Model file for the job. Use its own axes, mm. Coordinates: 2 decimals unless noted, no trailing zeros. Order: outer loops, then holes, each group sorted by start corner. A loop starts at its lowest first (then second) coordinate and runs counter-clockwise, first axis right, second up. Notation, with made-up numbers: (-20, 23) -> (39, 23) arc R22 ccw to (39, 30) -> close; hole circle Ø6 at (31.25, -22.5). An arc over 180 degrees is marked (long way). Write item = value, one per line. Start each with the question number.
Q1. Cut at A-A, the plane y = 35. List the corners of the cut face in (x, z).
Q2. Cut at C-C, the plane x = 130. List the corners of the cut face in (y, z), plus the area to 3 significant figures.
Q3. Wall check: line 1 (X direction, y = 34.5, z = 0.45); line 2 (X direction, y = 31, z = 0.95); line 3 (Y direction, x = 130, z = 1.3). Give the ranges that are in metal, low to high. Write a range as from..to.
Q4. Flat gauge pins, fed straight in: pin 1 (12 mm diameter, centred on x = 40, y = 35, fed in from -Z); pin 2 (2 mm diameter, centred on x = 23, z = 2, fed in from +Y); pin 3 (2 mm diameter, centred on y = 70.5, z = 2.5, fed in from -X); pin 4 (1.2 mm diameter, centred on y = 12, z = 1, fed in from -X). Where does each tip first touch, or does it go through?
Q5. Cut at B-B, the plane z = 3.4. List the corners of the cut face in (x, y), plus the area to 3 significant figures.
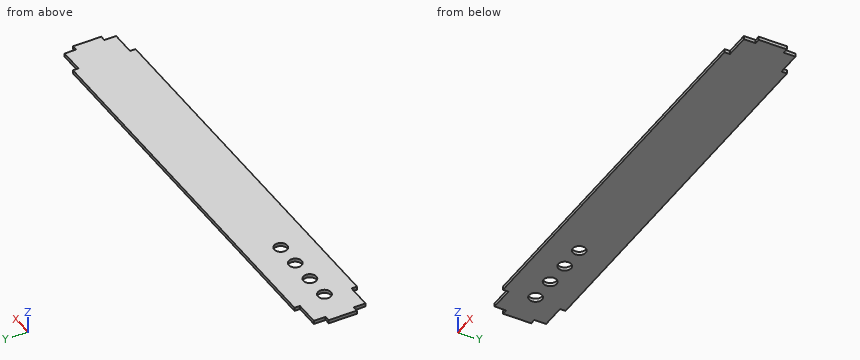
Autodesk Inventor part; units mm, degrees
ref_plane "YZ Plane" through (0, 0, 0) normal (1, 0, 0) x (0, 1, 0)
ref_plane "XZ Plane" through (0, 0, 0) normal (0, 1, 0) x (-1, 0, 0)
ref_plane "XY Plane" through (0, 0, 0) normal (0, 0, 1) x (1, 0, 0)
sketch "Skizze1" plane through (0, 0, 0) normal (0, 0, 1) x (1, 0, 0)
  line L0 (0, 0) -> (526.5, 0)
  line L1 (526.5, 0) -> (526.5, 72.5)
  line L2 (526.5, 72.5) -> (0, 72.5)
  line L3 (0, 72.5) -> (0, 0)
  line L4 (0, 72.5) -> (35, 72.5)
  line L5 (35, 72.5) -> (35, 66.15)
  line L6 (35, 66.15) -> (0, 66.15)
  line L7 (0, 66.15) -> (0, 72.5)
  line L8 (0, 72.5) -> (6.35, 72.5)
  line L9 (6.35, 72.5) -> (6.35, 52.5)
  line L10 (6.35, 52.5) -> (0, 52.5)
  line L11 (0, 52.5) -> (0, 72.5)
  line L12 (0, 36.25) -> (526.5, 36.25) construction
  line L13 (263.25, 72.5) -> (263.25, 0) construction
  line L14 (0, 0) -> (35, 0)
  line L15 (35, 0) -> (35, 6.35)
  line L16 (35, 6.35) -> (0, 6.35)
  line L17 (0, 6.35) -> (0, 0)
  line L18 (0, 0) -> (6.35, 0)
  line L19 (6.35, 0) -> (6.35, 20)
  line L20 (6.35, 20) -> (0, 20)
  line L21 (0, 20) -> (0, 0)
  line L22 (526.5, 72.5) -> (526.5, 0)
  line L23 (526.5, 72.5) -> (491.5, 72.5)
  line L24 (491.5, 72.5) -> (491.5, 66.15)
  line L25 (491.5, 66.15) -> (526.5, 66.15)
  line L26 (526.5, 66.15) -> (526.5, 72.5)
  line L27 (526.5, 72.5) -> (520.15, 72.5)
  line L28 (520.15, 72.5) -> (520.15, 52.5)
  line L29 (520.15, 52.5) -> (526.5, 52.5)
  line L30 (526.5, 52.5) -> (526.5, 72.5)
  line L31 (526.5, 0) -> (520.15, 0)
  line L32 (526.5, 0) -> (491.5, 0)
  line L33 (491.5, 0) -> (491.5, 6.35)
  line L34 (491.5, 6.35) -> (526.5, 6.35)
  line L35 (520.15, 0) -> (520.15, 20)
  line L36 (526.5, 6.35) -> (526.5, 0)
  line L37 (520.15, 20) -> (526.5, 20)
  line L38 (526.5, 20) -> (526.5, 0)
  point P0 (520.15, 66.15)
  point P1 (6.35, 66.15)
  point P2 (0, 52.5)
  point P3 (0, 20)
  point P4 (6.35, 6.35)
  point P5 (491.5, 0)
  point P6 (520.15, 6.35)
  point P7 (526.5, 20)
  dimension "d0" = 526.5
  dimension "d1" = 72.5
  dimension "d2" = 35
  dimension "d3" = 6.35
  dimension "d4" = 6.35
  dimension "d5" = 20
extrude "Extrusion1" add sketch "Skizze1" along normal blind 4 contours L15 L16 L19 L20 L3 L10 L9 L6 L5 L2 L24 L25 L28 L29 L1 L37 L35 L34 L33 L0
sketch "Skizze2" plane through (0, 0, 4) normal (0, 0, 1) x (1, 0, 0)
  circle A0 centre (40, 35) radius 7.5
  circle A1 centre (70, 35) radius 7.5
  circle A2 centre (100, 35) radius 7.5
  circle A3 centre (130, 35) radius 7.5
  line L0 (35, 0) -> (491.5, 0)
  line L1 (0, 52.5) -> (0, 20)
  point P0 (0, 0)
  dimension "d8" = 15
  dimension "d9" = 15
  dimension "d10" = 15
  dimension "d11" = 15
  dimension "d12" = 35
  dimension "d13" = 30
  dimension "d14" = 40
  dimension "d15" = 30
  dimension "d16" = 30
extrude "Extrusion2" cut sketch "Skizze2" against normal blind 10
properties part number "103.013.01_Abdeckung_Gestell_hinten" material "PMMA-Kunststoff"
Here are the results:
q1.outline = (0, 0) -> (32.5, 0) -> (32.5, 4) -> (0, 4) -> close; (47.5, 0) -> (62.5, 0) -> (62.5, 4) -> (47.5, 4) -> close; (77.5, 0) -> (92.5, 0) -> (92.5, 4) -> (77.5, 4) -> close; (107.5, 0) -> (122.5, 0) -> (122.5, 4) -> (107.5, 4) -> close; (137.5, 0) -> (526.5, 0) -> (526.5, 4) -> (137.5, 4) -> close
q2.outline = (0, 0) -> (27.5, 0) -> (27.5, 4) -> (0, 4) -> close; (42.5, 0) -> (72.5, 0) -> (72.5, 4) -> (42.5, 4) -> close
q2.area = 230 mm²
q3.line_1 = 0..32.52, 47.48..62.52, 77.48..92.52, 107.48..122.52, 137.48..526.5
q3.line_2 = 0..33.66, 46.34..63.66, 76.34..93.66, 106.34..123.66, 136.34..526.5
q3.line_3 = 0..27.5, 42.5..72.5
q4.pin_1 = through
q4.pin_2 = 66.15
q4.pin_3 = 35
q4.pin_4 = 6.35
q5.outline = (0, 20) -> (6.35, 20) -> (6.35, 6.35) -> (35, 6.35) -> (35, 0) -> (491.5, 0) -> (491.5, 6.35) -> (520.15, 6.35) -> (520.15, 20) -> (526.5, 20) -> (526.5, 52.5) -> (520.15, 52.5) -> (520.15, 66.15) -> (491.5, 66.15) -> (491.5, 72.5) -> (35, 72.5) -> (35, 66.15) -> (6.35, 66.15) -> (6.35, 52.5) -> (0, 52.5) -> close; hole circle Ø15 at (40, 35); hole circle Ø15 at (70, 35); hole circle Ø15 at (100, 35); hole circle Ø15 at (130, 35)
q5.area = 36,200 mm²
